from build123d import *

# Parameters (mm, degrees)
SKETCH1_R           = 15
BOSS_EXTRUDE1_DEPTH = 3
BOSS_EXTRUDE5_DEPTH = 30
BOSS_EXTRUDE6_START = 3
SKETCH5_R           = 15
BOSS_EXTRUDE6_DEPTH = 3
CUT_EXTRUDE1_DEPTH  = 242.0136151


with BuildPart() as part:
    # Sketch1 → Boss-Extrude1 (new body)
    with BuildSketch(Plane(origin=(0, 0, 0), x_dir=(1, 0, 0), z_dir=(0, 1, 0))):
        with BuildLine():
            Line((-10, 167.320508076), (-10, 17.320508076))
            ThreePointArc((-10, 17.320508076), (0, -20), (10, 17.320508076))
            Line((10, 17.320508076), (10, 167.320508076))
            ThreePointArc((10, 167.320508076), (0, 177.320508076), (-10, 167.320508076))
        make_face()
        with Locations(Location((0, 0, 0), (0, 0, 270))):
            Circle(SKETCH1_R, mode=Mode.SUBTRACT)
    extrude(amount=BOSS_EXTRUDE1_DEPTH)

    # Sketch4 → Boss-Extrude5 (add)
    with BuildSketch(Plane(origin=(0, 0, -177.320508076), x_dir=(-1, 0, 0), z_dir=(0, 0, -1))):
        with BuildLine():
            Line((0, 0), (0, 3))
            ThreePointArc((0, 3), (70, 73), (0, 143))
            Line((0, 143), (0, 146))
            ThreePointArc((0, 146), (73, 73), (0, 0))
        make_face()
    extrude(amount=-BOSS_EXTRUDE5_DEPTH)

    # Sketch5 → Boss-Extrude6 (add)
    with BuildSketch(Plane(origin=(0, 146, 0), x_dir=(-1, 0, 0), z_dir=(0, -1, 0)).offset(BOSS_EXTRUDE6_START)):
        with BuildLine():
            Line((10, 17.320508076), (10, 167.320508076))
            ThreePointArc((10, 167.320508076), (0, 177.320508076), (-10, 167.320508076))
            Line((-10, 167.320508076), (-10, 17.320508076))
            ThreePointArc((-10, 17.320508076), (0, -20), (10, 17.320508076))
        make_face()
        with Locations(Location((0, 0, 0), (0, 0, 270))):
            Circle(SKETCH5_R, mode=Mode.SUBTRACT)
    extrude(amount=-BOSS_EXTRUDE6_DEPTH)

    # Sketch7 → Cut-Extrude1 (cut, through all)
    with BuildSketch(Plane(origin=(0, 146, 0), x_dir=(1, 0, 0), z_dir=(0, 1, 0))):
        with BuildLine():
            Line((0.5, 152.804939292), (-0.5, 152.804939292))
            ThreePointArc((-0.5, 152.804939292), (-1.914213562, 153.39072573), (-2.5, 154.804939292))
            Line((-2.5, 154.804939292), (-2.5, 170.804939292))
            ThreePointArc((-2.5, 170.804939292), (-1.914213562, 172.219152855), (-0.5, 172.804939292))
            Line((-0.5, 172.804939292), (0.5, 172.804939292))
            ThreePointArc((0.5, 172.804939292), (1.914213562, 172.219152855), (2.5, 170.804939292))
            Line((2.5, 170.804939292), (2.5, 154.804939292))
            ThreePointArc((2.5, 154.804939292), (1.914213562, 153.39072573), (0.5, 152.804939292))
        make_face()
        with BuildLine():
            Line((0.5, 65.676892474), (-0.5, 65.676892474))
            ThreePointArc((-0.5, 65.676892474), (-1.914213562, 66.262678911), (-2.5, 67.676892474))
            Line((-2.5, 67.676892474), (-2.5, 83.676892474))
            ThreePointArc((-2.5, 83.676892474), (-1.914213562, 85.091106036), (-0.5, 85.676892474))
            Line((-0.5, 85.676892474), (0.5, 85.676892474))
            ThreePointArc((0.5, 85.676892474), (1.914213562, 85.091106036), (2.5, 83.676892474))
            Line((2.5, 83.676892474), (2.5, 67.676892474))
            ThreePointArc((2.5, 67.676892474), (1.914213562, 66.262678911), (0.5, 65.676892474))
        make_face()
    extrude(amount=-CUT_EXTRUDE1_DEPTH, mode=Mode.SUBTRACT)


solid = part.part
For this review, take the finished solid that the model builds, in its own axes (mm). A direction names the side the tool comes from. Give positions to 0.01 mm unless a question says otherwise; leave off trailing zeros. Order: outer loops, then holes, each group sorted by start corner. A loop starts at its lowest first (then second) coordinate and runs counter-clockwise, first axis right, second up. Notation, with made-up numbers: M 12.5,16 L 42.5,16 A10 cw 42.5,32 Z; hole C 36.5,8 d7. An arc over 180 degrees is marked long. Answer in a Markdown table with one row per item. Add a question column.
(1) Consider section B-B on x = -31. State the section outline as (y, z) points, and give its area (3 significant figures).
(2) Consider section D-D on y = 73. State the section outline as (x, z) points, and give its area (3 significant figures).
(3) Consider section C-C on x = -54.5. State the section outline as (y, z) points, and give its area (3 significant figures).
(4) For pin 1 (0.9 mm diameter, centred on y = 144, z = -58.5, fed in from +X); pin 2 (2.5 mm diameter, centred on y = 1, z = -72, fed in from -X), all flat-tipped, find the tip position at first contact; note any pin that passes through.
(5) Consider section A-A on z = 0. State the section outline as (x, y) points, and give its area (3 significant figures).
(6) Wall thickness on probe 1 along X at (y, z) = (0.8, 0); probe 2 along Y at (x, z) = (-1.5, -40); probe 3 along Y at (x, z) = (-20.5, -157): over which ranges is each line inside the solid? List them lowest first. Write a range as [from, to].
(7) For faces 1 (the face through (7.15, 1.48, -174.31)), 2 (the face through (-9.016, 0.263, -171.646)), 3 (the face through (-72.982, 74.605, -162.531)), list the 3-axis set-ups (+Z, -Z, +X, -X, +Y, -Y) from which the entire face can be reached by the end or side of a thin tool; tool diameter is ignored.
(8) Mouldability with a two-part tool opening along X and no side actions: class faces 4 (the face through (0.733, 144.479, 19.987)), 5 (the face through (-0.66, 144.479, -14.985)), 6 (the face through (-9.109, 145.728, -171.447)), 7 (the face through (-69, 89, -147.321)) as +X half, -X half, draft (parallel to the pull), parting line (faces both ways), or undercut.
Evaluation:
| question | item | result |
|---|---|---|
| 1 | outline | M 6.91,-177.32 L 10.24,-177.32 L 10.24,-147.32 L 6.91,-147.32 Z; M 135.76,-177.32 L 139.09,-177.32 L 139.09,-147.32 L 135.76,-147.32 Z |
| 1 | area | 200 mm^2 |
| 2 | outline | M -73,-177.32 L -70,-177.32 L -70,-147.32 L -73,-147.32 Z |
| 2 | area | 90.0 mm^2 |
| 3 | outline | M 24.43,-177.32 L 29.07,-177.32 L 29.07,-147.32 L 24.43,-147.32 Z; M 116.93,-177.32 L 121.57,-177.32 L 121.57,-147.32 L 116.93,-147.32 Z |
| 3 | area | 278 mm^2 |
| 4 | pin 1 | stops at x = 10 |
| 4 | pin 2 | stops at x = -10 |
| 5 | outline | M -20,0 L -15,0 L -15,3 L -20,3 Z; M -20,143 L -15,143 L -15,146 L -20,146 Z; M 15,0 L 20,0 L 20,3 L 15,3 Z; M 15,143 L 20,143 L 20,146 L 15,146 Z |
| 5 | area | 60.0 mm^2 |
| 6 | probe 1 | x = [-20, -15], [15, 20] |
| 6 | probe 2 | y = [0, 3], [143, 146] |
| 6 | probe 3 | y = [2.94, 6.07], [139.93, 143.06] |
| 7 | face 1 | -Z, +X, +Y, -Y |
| 7 | face 2 | -Z, -X, -Y |
| 7 | face 3 | -Z, -X |
| 8 | face 4 | parting line |
| 8 | face 5 | undercut |
| 8 | face 6 | -X half |
| 8 | face 7 | draft |
